Solid Edge part; units mm, degrees
sketch "Sketch1" plane through (0, 0, 0) normal (0, 0, 1) x (1, 0, 0)
  circle A0 centre (0, 0) radius 2.8702
extrude "Protrusion1" add sketch "Sketch1" along normal blind 3.5052
sketch "Sketch2" plane through (0, 0, 0) normal (0, 0, -1) x (1, 0, 0)
  circle A0 centre (0, 0) radius 1.7526
extrude "Protrusion2" add sketch "Sketch2" along normal blind 25.4
sketch "Sketch3" plane through (0, 0, -25.4) normal (0, 0, -1) x (1, 0, 0)
  circle A0 centre (0, 0) radius 1.7523
extrude "Cutout1" cut sketch "Sketch3" against normal blind 17.4625 flip side to cut
chamfer "Chamfer_1" distance 0.2629 angle 45 1 edges at (-1.7523, 0, -25.4)
sketch "Sketch4" plane through (0, 0, 3.5052) normal (0, 0, 1) x (1, 0, 0)
  line L0 (-0.802, 1.3891) -> (0.802, 1.3891)
  line L1 (1.604, 0) -> (0.802, 1.3891)
  line L2 (0.802, -1.3891) -> (1.604, 0)
  line L3 (-0.802, -1.3891) -> (0.802, -1.3891)
  line L4 (-1.604, 0) -> (-0.802, -1.3891)
  line L5 (-0.802, 1.3891) -> (-1.604, 0)
extrude "Cutout2" cut sketch "Sketch4" against normal blind 1.7526
properties part number "24101587"
Could you check a few things on this model? Use its own coordinates, in mm. A direction names the side the tool comes from. Coordinates: 2 decimals unless noted, no trailing zeros. Write each loop counter-clockwise with the first axis right and the second up, starting at its lowest first coordinate (ties: lowest second). Pieces come first, ordered by that corner, then holes. Notation, with made-up numbers: (35.5, 74.25) -> (91.5, 74.25) arc R22 ccw to (91.5, 98.25) -> close; hole circle Ø8 at (25.25, 67.25). An arc over 180 degrees is marked (long way). One line per question, with ' | ' between items. Start each with the question number.
1. Thinking about a two-plate mould opening in Y: for faces 1 (the face through (1.2, 0.7, 2.6)), 2 (the face through (1.67, 0.53, -3.91)), 3 (the face through (0, -2, 0)), which applies, pulls with the +Y half, pulls with the -Y half, needs draft (parallel to the pull), parting line crosses it, or undercut?
2. Will these pins go through, and if not, where does the flat tip stop? P1, Ø3, axis at y = 0, z = -12, coming from the -X side; P2, Ø3, axis at x = -2, z = -21.5, coming from the +Y side; P3, Ø1, axis at x = -2, z = -19, coming from the -Y side.
3. If we section it at C-C (y = 2.4): Please give me the cut outline in (x, z).
4. If we section it at D-D (x = -2): Please give me the cut outline in (y, z), and give its area (3 significant figures).
5. Please list where these lines run through material, in increasing order: line 1 along Z through (x, y) = (2.2, -1.15); line 2 along Y through (x, z) = (0, -23.5); line 3 along Y through (x, z) = (-0.7, -4.25).
6. If we section it at B-B (z = -13.5): Please give me the cut outline in (x, y).
7. For faces 4 (the face through (1.67, -0.53, -16.66)), 5 (the face through (-2.278, 1.746, 1.728)), 6 (the face through (-1.2, -0.7, 2.6)), which set-ups out of +Z, -Z, +X, -X, +Y, -Y let a thin tool reach every point of the face, with its end or its side?
Return value:
1) face 1: undercut | face 2: parting line crosses it | face 3: needs draft
2) P1: stops at x = -1.75 | P2: stops at y = 1.68 | P3: stops at y = -0.91
3) outline: (-1.57, 0) -> (1.57, 0) -> (1.57, 3.51) -> (-1.57, 3.51) -> close
4) outline: (-2.06, 0) -> (2.06, 0) -> (2.06, 3.51) -> (-2.06, 3.51) -> close | area: 14.4 mm²
5) line 1: z = 0 to 3.51 | line 2: y = -1.75 to 1.75 | line 3: y = -1.61 to 1.61
6) outline: circle Ø3.5 at (0, 0)
7) face 4: -Z | face 5: +Z, -Z | face 6: +Z
